CAD build for the part. Positions are in the model's coordinates, mm. A direction names the side the tool comes from. Coordinates: 2 decimals unless noted, no trailing zeros. Order: outer loops, then holes, each group sorted by start corner. A loop starts at its lowest first (then second) coordinate and runs counter-clockwise, first axis right, second up. Notation, with made-up numbers: M -40,8.25 L 5,8.25 A19 ccw 5,26.25 Z; hole C 79,-28 d1. An arc over 180 degrees is marked long. One line per item, written item: value.
from build123d import *

# Parameters (mm, degrees)
F0_W     = 8
F0_H     = 16
F1_DEPTH = 10
F2_R     = 2.5
F3_DEPTH = 1
F4_T     = -1.5
F6_DEPTH = 10


with BuildPart() as f1:
    # F0 (on Top) → F1 (new body)
    with BuildSketch(Plane.XY):
        with Locations((-6.5223464929, 11.4436195551)):
            Rectangle(F0_W, F0_H)
    extrude(amount=F1_DEPTH)

    # F2 (on face) → F3 (join)
    with BuildSketch(Plane.XY.offset(10)):
        with Locations((-6.5223464929, 7.4436195551)):
            Circle(F2_R)
        with Locations((-6.5223464929, 15.4436195551)):
            Circle(F2_R)
    extrude(amount=F3_DEPTH)

    # F4
    f4_openings = [f1.faces().sort_by_distance(p)[0] for p in [
        (-6.522346, 11.44362, 0),
    ]]
    offset(amount=F4_T, openings=f4_openings, kind=Kind.INTERSECTION)

    # F5 (on face) → F6 (join)
    with BuildSketch(Plane.XY.offset(10)):
        with BuildLine():
            ThreePointArc((-6.5223464929, 9.9436195551), (-5.4616863211, 10.3829593833), (-5.0223464929, 11.4436195551))
            ThreePointArc((-5.0223464929, 11.4436195551), (-5.4616863203, 12.5042797261), (-6.5223464908, 12.9436195551))
            ThreePointArc((-6.5223464908, 12.9436195551), (-8.0223464929, 11.4436195561), (-6.5223464929, 9.9436195551))
        make_face()
    extrude(amount=-F6_DEPTH)


solid = f1.part
Q1. Slice it at D-D (z = 8.75). List the corners of the cut face in (x, y).
Recorded:
outline: M -10.52,3.44 L -2.52,3.44 L -2.52,19.44 L -10.52,19.44 Z; hole C -6.52,7.44 d2; hole C -6.52,15.44 d2
Q2. Slice it at A-A (z = 6.5). List the corners of the cut face in (x, y).
Recorded:
outline: M -10.52,3.44 L -2.52,3.44 L -2.52,19.44 L -10.52,19.44 Z; C -6.52,11.44 d3; hole M -9.02,4.94 L -4.02,4.94 L -4.02,17.94 L -9.02,17.94 Z
Q3. Pin check, flat tips, straight feed: pin 1 Ø4 at (x, y) = (-6.5, 12) entering from -Z; pin 2 Ø2 at (x, y) = (-6.5, 7.5) entering from -Z. Stop position of each tip, or through.
Recorded:
pin 1: stops at z = 0
pin 2: stops at z = 8.5
Q4. Slice it at B-B (x = -4.5). List the corners of the cut face in (y, z), plus the area to 3 significant figures.
Recorded:
outline: M 3.44,0 L 4.94,0 L 4.94,8.5 L 17.94,8.5 L 17.94,0 L 19.44,0 L 19.44,10 L 16.91,10 L 16.91,11 L 13.97,11 L 13.97,10 L 8.91,10 L 8.91,11 L 5.97,11 L 5.97,10 L 3.44,10 Z
area: 55.4 mm^2
Q5. Slice it at C-C (y = 17). List the corners of the cut face in (x, z), plus the area to 3 significant figures.
Recorded:
outline: M -10.52,0 L -9.02,0 L -9.02,8.5 L -4.02,8.5 L -4.02,0 L -2.52,0 L -2.52,10 L -4.57,10 L -4.57,11 L -8.48,11 L -8.48,10 L -10.52,10 Z
area: 41.4 mm^2
Q6. Drill centre lines: line 1 along X through (y, z) = (16.5, 2.25); line 2 along X through (y, z) = (12.5, 1.25); line 3 along Y through (x, z) = (-4.5, 8). Where is each one in solid material? Low to high.
Recorded:
line 1: x = -10.52 to -9.02, -4.02 to -2.52
line 2: x = -10.52 to -9.02, -7.59 to -5.46, -4.02 to -2.52
line 3: y = 3.44 to 4.94, 17.94 to 19.44
Q7. Which spindle directions (+Z, -Z, +X, -X, +Y, -Y) get a long thin tool onto all of the face, cutting with end or side? Do faces 1 (the face through (-4.022, 11, 4)), 2 (the face through (-7, 12, 10)), 3 (the face through (-7, 19.444, 5)). Say none if no direction does.
Recorded:
face 1: -Z
face 2: +Z
face 3: +Z, -Z, +X, -X, +Y
